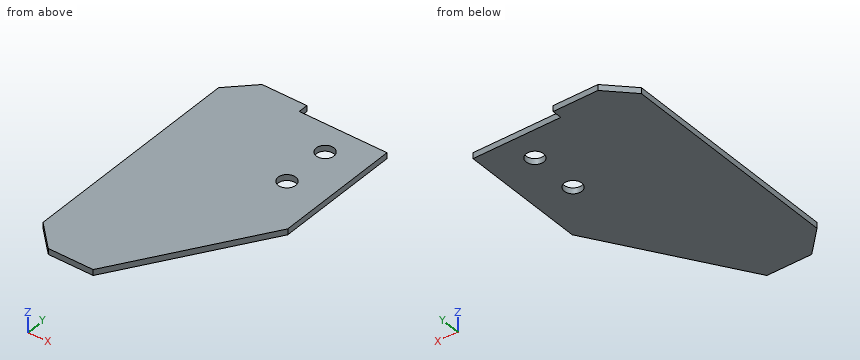
Autodesk Fusion 360 part; units mm, degrees
sketch "スケッチ1" plane through (0, 0, 0) normal (0, 0, 1) x (1, 0, 0)
  line L0 (-9.5, 140) -> (-80.5, 140)
  line L1 (-80.5, 140) -> (-80.5, -140)
  line L2 (-80.5, -140) -> (-9.5, -140)
  line L3 (80.5, 0) -> (80.5, 130)
  line L4 (74.75, 130) -> (-80.5, -140) construction
  line L5 (-80.5, 140) -> (38.0073, -66.0997) construction
  line L6 (-9.5, 140) -> (-9.5, 130)
  line L7 (-9.5, 130) -> (80.5, 130)
  line L8 (-80.5, -140) -> (-9.5, -140) construction
  line L9 (80.5, 0) -> (-9.5, -140)
  dimension "d2" = 280
  dimension "d5" = 71
extrude "押し出し1" add sketch "スケッチ1" along normal blind 6
chamfer "面取り1" distance 25 angle 45 2 edges at (-80.5, -140, 3) (-80.5, 140, 3)
sketch "スケッチ2" plane through (0, 0, 6) normal (0, 0, 1) x (-1, 0, 0)
  line L0 (55.5, -140) -> (80.5, -115)
  line L1 (80.5, -115) -> (80.5, 115)
  line L2 (80.5, 115) -> (55.5, 140)
  line L3 (55.5, 140) -> (9.5, 140)
  line L4 (9.5, 140) -> (-80.5, 0)
  line L5 (-80.5, 0) -> (-80.5, -130)
  line L6 (-80.5, -130) -> (9.5, -130)
  line L7 (9.5, -130) -> (9.5, -140)
  line L8 (9.5, -140) -> (55.5, -140)
  line L9 (-80.5, -130) -> (-40.5, -130) construction
  line L10 (-40.5, -130) -> (-40.5, -100) construction
  line L11 (-40.5, -100) -> (-80.5, -100) construction
  line L12 (-80.5, -100) -> (-80.5, -130) construction
  line L13 (-40.5, -100) -> (-40.5, -50) construction
  point P0 (-40.5, -100)
  point P1 (-40.5, -50)
  dimension "d10" = 40
  dimension "d11" = 30
  dimension "d12" = 50
hole "穴1" at (40.5, 100, 6) at (40.5, 50, 6) direction (0, 0, -1) diameter 18 end through all
equation "d5 = 25 mm + 46 mm"
Model file for the job. Use its own axes, mm. Round coordinates to 2 decimals unless told otherwise and drop trailing zeros. Loops run counter-clockwise (first coordinate to the right, second up) from the corner with the lowest first, then second, coordinate; pieces in that order, holes last.
1. Band-saw the part on A-A, the plane y = 100.5. List the corners of the cut face in (x, z), and give its area (3 significant figures).
Check values:
outline: (-80.5, 0) - (31.51, 0) - (31.51, 6) - (-80.5, 6) - close; (49.49, 0) - (80.5, 0) - (80.5, 6) - (49.49, 6) - close
area: 858 mm2
2. Wall check: probe 1 along X at (y, z) = (50, 3.65); probe 2 along Y at (x, z) = (40.5, 3.9); probe 3 along Y at (x, z) = (41.5, 5.25). Give the ranges that are in metal, low to high.
Check values:
probe 1: x = -80.5 to 31.5, 49.5 to 80.5
probe 2: y = -62.22 to 41, 59 to 91, 109 to 130
probe 3: y = -60.67 to 41.06, 58.94 to 91.06, 108.94 to 130
3. Band-saw the part on D-D, the plane y = 50. List the corners of the cut face in (x, z), and give its area (3 significant figures).
Check values:
outline: (-80.5, 0) - (31.5, 0) - (31.5, 6) - (-80.5, 6) - close; (49.5, 0) - (80.5, 0) - (80.5, 6) - (49.5, 6) - close
area: 858 mm2
4. Drop a flat-ended pin along its axis: P1, Ø1.5, axis at x = 0, z = 3, coming from the +Y side. Give the stop position or say it passes through.
Check values:
P1: stops at y = 130
5. Band-saw the part on B-B, the plane z = 4.65. List the corners of the cut face in (x, y).
Check values:
outline: (-80.5, -115) - (-55.5, -140) - (-9.5, -140) - (80.5, 0) - (80.5, 130) - (-9.5, 130) - (-9.5, 140) - (-55.5, 140) - (-80.5, 115) - close; hole circle Ø18 at (40.5, 50); hole circle Ø18 at (40.5, 100)
6. Band-saw the part on C-C, the plane x = 40.5. List the corners of the cut face in (y, z).
Check values:
outline: (-62.22, 0) - (41, 0) - (41, 6) - (-62.22, 6) - close; (59, 0) - (91, 0) - (91, 6) - (59, 6) - close; (109, 0) - (130, 0) - (130, 6) - (109, 6) - close
